The listing builds one solid part. Answer for the finished solid, in the listing's coordinates (mm). A direction names the side the tool comes from. Round coordinates to 2 decimals unless told otherwise and drop trailing zeros. Write each loop counter-clockwise with the first axis right and the second up, starting at its lowest first coordinate (ties: lowest second). Pieces come first, ordered by that corner, then holes.
(1) The mould has two halves that part along X. Classify faces 3 (the face through (-101.6, 0, 0)), 4 (the face through (-50.267, -24.796, 5.506)), 5 (the face through (457.2, 0, 0)), 6 (the face through (447.004, -30.995, 6.883)): +X half, -X half, draft (parallel to the pull), parting line (faces both ways), or undercut.
(2) Each of these flat-tipped pins is pushed along its axis until it touches: pin 1 Ø3 at (x, z) = (165.5, -2) entering from +Y; pin 2 Ø1 at (y, z) = (18.5, 16.5) entering from -X; pin 3 Ø8 at (x, y) = (320.5, -9.5) entering from +Z; pin 4 Ø2 at (y, z) = (-6.5, 24) entering from +X. Where does it stop, or does it pass through?
(3) Find the intervals of material crossed by probe 1 along X at (y, z) = (-24, 8.5); probe 2 along X at (y, z) = (20.5, 20); probe 3 along Y at (x, z) = (296, 0.5), in increasing order.
(4) For faces 1 (the face through (355.6, 21.3, 14.3)), 2 (the face through (361.861, -30.995, 6.883)), determine the directions among +Z, -Z, +X, -X, +Y, -Y from which every point of the face is accessible in a straight line to the end or side of a thin tool.
(5) A cutting plane is placed at D-D, the plane x = 361.5. Give the vertices of the cut face in (y, z).
(6) A cutting plane is placed at C-C, the plane x = 297. Give the vertices of the cut face in (y, z), and give its area (3 significant figures).
from build123d import *

# Parameters (mm, degrees)
SKETCH1_R           = 25.4
BOSS_EXTRUDE1_DEPTH = 355.6
SKETCH2_R           = 31.75
BOSS_EXTRUDE2_DEPTH = 12.7
SKETCH3_R           = 25.4
BOSS_EXTRUDE3_DEPTH = 76.2
SKETCH4_R           = 31.75
BOSS_EXTRUDE4_DEPTH = 12.7
FILLET1_R           = 7.62
FILLET2_R           = 7.62


with BuildPart() as part:
    # Sketch1 → Boss-Extrude1 (new body)
    with BuildSketch(Plane(origin=(0, 0, 0), x_dir=(0, 0, -1), z_dir=(1, 0, 0))):
        Circle(SKETCH1_R)
    extrude(amount=BOSS_EXTRUDE1_DEPTH)

    # Sketch2 → Boss-Extrude2 (add)
    with BuildSketch(Plane(origin=(355.6, 0, 0), x_dir=(0, 0, -1), z_dir=(1, 0, 0))):
        Circle(SKETCH2_R)
    boss_extrude2 = extrude(amount=BOSS_EXTRUDE2_DEPTH)

    # Sketch3 → Boss-Extrude3 (add)
    with BuildSketch(Plane(origin=(368.3, 0, 0), x_dir=(0, 0, -1), z_dir=(1, 0, 0))):
        Circle(SKETCH3_R)
    boss_extrude3 = extrude(amount=BOSS_EXTRUDE3_DEPTH)

    # Sketch4 → Boss-Extrude4 (add)
    with BuildSketch(Plane(origin=(444.5, 0, 0), x_dir=(0, 0, -1), z_dir=(1, 0, 0))):
        Circle(SKETCH4_R)
    boss_extrude4 = extrude(amount=BOSS_EXTRUDE4_DEPTH)

    # Mirror1: Boss-Extrude2, Boss-Extrude3, Boss-Extrude4 across plane
    add(boss_extrude2.mirror(Plane.ZY.offset(-177.8)))
    add(boss_extrude3.mirror(Plane.ZY.offset(-177.8)))
    add(boss_extrude4.mirror(Plane.ZY.offset(-177.8)))

    # Fillet1
    fillet1_edges = [part.edges().sort_by_distance(p)[0] for p in [
        (457.2, 0, 31.75),
    ]]
    fillet(fillet1_edges, radius=FILLET1_R)

    # Fillet2
    fillet2_edges = [part.edges().sort_by_distance(p)[0] for p in [
        (-101.6, 0, 31.75),
    ]]
    fillet(fillet2_edges, radius=FILLET2_R)


solid = part.part
Solutions:
1. face 3: -X half
1. face 4: undercut
1. face 5: +X half
1. face 6: draft
2. pin 1: stops at y = 25.4
2. pin 2: stops at x = -101.6
2. pin 3: stops at z = 24.8
2. pin 4: stops at x = 457.2
3. probe 1: x = -101.48 to -88.9, -12.7 to 0, 355.6 to 368.3, 444.5 to 457.08
3. probe 2: x = -100.12 to -88.9, -12.7 to 0, 355.6 to 368.3, 444.5 to 455.72
3. probe 3: y = -25.4 to 25.4
4. face 1: none
4. face 2: +X, -X
5. outline: circle Ø63.5 at (0, 0)
6. outline: circle Ø50.8 at (0, 0)
6. area: 2,030 mm2
